from build123d import *

# Parameters (mm, degrees)
SKETCH1_R           = 3.0988
BOSS_EXTRUDE1_DEPTH = 12.7
BOSS_EXTRUDE2_DEPTH = 21.59


with BuildPart() as part:
    # Sketch1 → Boss-Extrude1 (new body)
    with BuildSketch(Plane.XY):
        Circle(SKETCH1_R)
    extrude(amount=-BOSS_EXTRUDE1_DEPTH)

    # Sketch2 → Boss-Extrude2 (add)
    with BuildSketch(Plane(origin=(0, 0, -12.7), x_dir=(-1, 0, 0), z_dir=(0, 0, -1))):
        Polygon((0, 3.666174209), (-3.175, 1.833087105), (-3.175, -1.833087105), (0, -3.666174209), (3.175, -1.833087105), (3.175, 1.833087105), align=None)
    extrude(amount=BOSS_EXTRUDE2_DEPTH)


solid = part.part
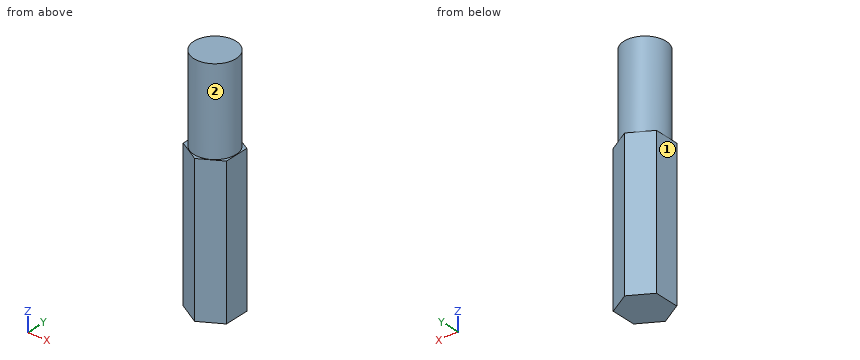
Here's how the part is built. I have some questions about the finished solid (model axes, mm). Face numbers are marked on the shaded views. A direction names the side the tool comes from. Coordinates: 2 decimals unless noted, no trailing zeros. Write each loop counter-clockwise with the first axis right and the second up, starting at its lowest first coordinate (ties: lowest second). Pieces come first, ordered by that corner, then holes.
1) If we section it at C-C (x = 2): List the corners of the cut face in (y, z) for me.
Filled in:
outline: (-2.51, -34.29) - (2.51, -34.29) - (2.51, -12.7) - (2.37, -12.7) - (2.37, 0) - (-2.37, 0) - (-2.37, -12.7) - (-2.51, -12.7) - close
2) I'm going to push flat-ended pins straight in: pin 1 (2 mm diameter, centred on x = 0.5, z = -16, fed in from +Y); pin 2 (3 mm diameter, centred on x = 2.5, y = -3, fed in from -Z); pin 3 (3 mm diameter, centred on y = -1, z = -7, fed in from -X); pin 4 (1.5 mm diameter, centred on x = 1, z = -14.5, fed in from -Y). Where does each tip first touch, or does it pass through?
Filled in:
pin 1: stops at y = 3.67
pin 2: stops at z = -34.29
pin 3: stops at x = -3.1
pin 4: stops at y = -3.52
3) Which directions (+Z, -Z, +X, -X, +Y, -Y) give clear straight access to the entire face, cutting with the end or side of a thin tool? Please do the marked faces 1 and 2.
Filled in:
face 1: +Z, -Z, -X, +Y, -Y
face 2: +Z
4) If I drill on line 1 (Y direction, x = -2.5, z = -4); line 2 (Y direction, x = 0.25, z = -22.5); line 3 (X direction, y = -0.75, z = -5.5), over which ranges is the centre line in solid material (lowest first)?
Filled in:
line 1: y = -1.83 to 1.83
line 2: y = -3.52 to 3.52
line 3: x = -3.01 to 3.01
5) If we section it at D-D (z = -8): List the corners of the cut face in (x, y) for me.
Filled in:
outline: circle Ø6.2 at (0, 0)
6) If we section it at B-B (y = -2.5): List the corners of the cut face in (x, z) for me.
Filled in:
outline: (-2.02, -34.29) - (2.02, -34.29) - (2.02, -12.7) - (1.83, -12.7) - (1.83, 0) - (-1.83, 0) - (-1.83, -12.7) - (-2.02, -12.7) - close
7) If we section it at A-A (z = -20.5): List the corners of the cut face in (x, y) for me (3 decimals).
Filled in:
outline: (-3.175, -1.833) - (0, -3.666) - (3.175, -1.833) - (3.175, 1.833) - (0, 3.666) - (-3.175, 1.833) - close
